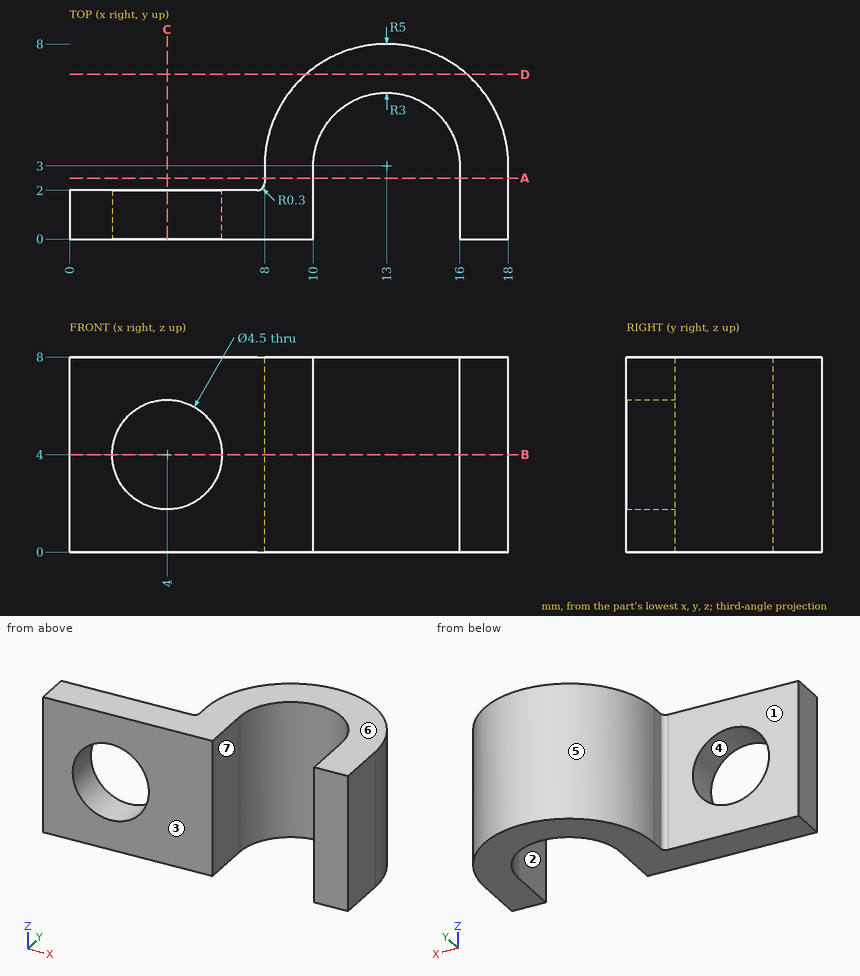
Study the drawing (mm; zero at the part's minimum x, y, z) and answer. A direction names the side the tool comes from. Give positions to 0.01 mm unless a question says otherwise; leave off trailing zeros. Write each loop counter-clockwise with the first axis right and the second up, starting at its lowest first coordinate (ties: lowest second). Pieces come first, ordered by that corner, then holes. Notation, with made-up numbers: (-17.75, -37) - (27.25, -37) arc R7 cw to (27.25, -29) - close; hole circle Ø1 at (50, 49.25). An arc over 180 degrees is marked (long way). Use a Markdown table: item, result.
1. Section B-B on z = 4 is taken. Write down the section's boundary in (x, y), plus the area to 3 significant figures.
Values follow:
| item | result |
|---|---|
| outline | (0, 0) - (1.75, 0) - (1.75, 2) - (0, 2) - close; (6.25, 0) - (10, 0) - (10, 3) arc R3 cw to (16, 3) - (16, 0) - (18, 0) - (18, 3) arc R5 ccw to (8, 3) - (8, 2.3) arc R0.3 cw to (7.7, 2) - (6.25, 2) - close |
| area | 44.2 mm² |
2. Section C-C on x = 4 is taken. Write down the section's boundary in (y, z), plus the area to 3 significant figures.
Values follow:
| item | result |
|---|---|
| outline | (0, 0) - (2, 0) - (2, 1.75) - (0, 1.75) - close; (0, 6.25) - (2, 6.25) - (2, 8) - (0, 8) - close |
| area | 7.00 mm² |
3. For a pull along X with two mould halves and no side action, classify the marked faces 4, 5, 6 and 7 as released by +X, released by -X, zero draft, split by the parting line, or undercut.
Values follow:
| item | result |
|---|---|
| face 4 | undercut |
| face 5 | split by the parting line |
| face 6 | zero draft |
| face 7 | undercut |
4. Section A-A on y = 2.5 is taken. Write down the section's boundary in (x, z), plus the area to 3 significant figures.
Values follow:
| item | result |
|---|---|
| outline | (8, 0) - (10, 0) - (10, 8) - (8, 8) - close; (16, 0) - (18, 0) - (18, 8) - (16, 8) - close |
| area | 32.0 mm² |
5. A tool of negligible diameter and unlimited length cuts with its end or side. For the marked faces 1, 2 and 3, from which of +Z, -Z, +X, -X, +Y, -Y can it reach the whole face along a straight path? Write none if from no direction.
Values follow:
| item | result |
|---|---|
| face 1 | +Z, -Z, -X, +Y |
| face 2 | +Z, -Z, -Y |
| face 3 | +Z, -Z, +X, -X, -Y |
6. Section D-D on y = 6.75 is taken. Write down the section's boundary in (x, z).
Values follow:
| item | result |
|---|---|
| outline | (9.69, 0) - (16.31, 0) - (16.31, 8) - (9.69, 8) - close |
7. Find the intervals of material crossed by probe 1 along Z at (x, y) = (4, 0.7); probe 2 along X at (y, z) = (2.25, 5.25); probe 3 along Y at (x, z) = (3, 1), in increasing order. Write a range as from..to.
Values follow:
| item | result |
|---|---|
| probe 1 | z = 0..1.75, 6.25..8 |
| probe 2 | x = 8..10, 16..18 |
| probe 3 | y = 0..2 |
